from build123d import *

# Parameters (mm, degrees)
F1_DEPTH = 3
F2_DEPTH = 22.5
F0_W     = 13.580743
F0_H     = 20.673372
F0_R     = 1.5
F3_DEPTH = 5


with BuildPart() as f1:
    # F0 (on Front) → F1 (new body)
    with BuildSketch(Plane.XZ):
        Polygon((26.088619, 25.064645), (26.088619, 26.396385), (-26.088619, 26.396385), (-26.088619, 25.064645), (-26.088619, -25.064645), (26.088619, -25.064645), align=None)
    extrude(amount=F1_DEPTH)

    # F0 (on Front) → F2 (join)
    with BuildSketch(Plane.XZ):
        Polygon((-27.5, -26.396385), (27.5, -26.396385), (27.5, -10.336686), (27.5, 10.336686), (27.5, 26.396385), (26.088619, 26.396385), (26.088619, 25.064645), (26.088619, -25.064645), (-26.088619, -25.064645), (-26.088619, 25.064645), (-26.088619, 26.396385), (-27.5, 26.396385), (-27.5, 10.336686), (-27.5, -10.336686), align=None)
    extrude(amount=F2_DEPTH)

    # F0 (on Front) → F3 (join)
    with BuildSketch(Plane.XZ):
        with Locations((-34.290371, 0)):
            Rectangle(F0_W, F0_H)
        with Locations((-34.290372, 0)):
            Circle(F0_R, mode=Mode.SUBTRACT)
        with Locations((34.290371, 0)):
            Rectangle(F0_W, F0_H)
        with Locations((34.290372, 0)):
            Circle(F0_R, mode=Mode.SUBTRACT)
    extrude(amount=F3_DEPTH)


solid = f1.part
Verification items for the finished model (mm, model axes). A direction names the side the tool comes from. Round coordinates to 2 decimals unless told otherwise and drop trailing zeros. Loops run counter-clockwise (first coordinate to the right, second up) from the corner with the lowest first, then second, coordinate; pieces in that order, holes last. Notation, with made-up numbers: (76.5, -14) - (89.5, -14) arc R31 cw to (89.5, 12) - close; hole circle Ø2 at (54, 69). An arc over 180 degrees is marked (long way). Use one line per item in the form item = value.
1. Access from +Z, -Z, +X, -X, +Y, -Y to the whole of each face (thin tool, end or side, straight path). Record for faces 4 (the flat face through (26.089, -13, 1)), 5 (the flat face through (34, -2, 10.337)), 6 (the flat face through (34, -5, 2)), 7 (the flat face through (-34, -2, 10.337)), 8 (the flat face through (-34, -2, -10.337)).
A:
face_4 = +Z, -Y
face_5 = +Z, +X, +Y, -Y
face_6 = +Z, -Z, +X, -Y
face_7 = +Z, -X, +Y, -Y
face_8 = -Z, -X, +Y, -Y
2. Section check C-C on x = 24. Record the cut outline in (y, z).
A:
outline = (-22.5, -26.4) - (0, -26.4) - (0, 26.4) - (-3, 26.4) - (-3, -25.06) - (-22.5, -25.06) - close
3. Section check A-A on z = 0. Record the cut outline in (x, y).
A:
outline = (-41.08, -5) - (-35.79, -5) - (-35.79, 0) - (-41.08, 0) - close; (-32.79, -5) - (-27.5, -5) - (-27.5, -22.5) - (-26.09, -22.5) - (-26.09, -3) - (26.09, -3) - (26.09, -22.5) - (27.5, -22.5) - (27.5, -5) - (32.79, -5) - (32.79, 0) - (-32.79, 0) - close; (35.79, -5) - (41.08, -5) - (41.08, 0) - (35.79, 0) - close
4. Scan lines: probe 1 along X at (y, z) = (-19.75, 16); probe 2 along X at (y, z) = (-2.75, 16); probe 3 along Z at (x, y) = (1.5, -18.5). Record each from-to range of solid material in increasing order.
A:
probe_1 = -27.5 to -26.09, 26.09 to 27.5
probe_2 = -27.5 to 27.5
probe_3 = -26.4 to -25.06
5. Section check D-D on z = 5.5. Record the cut outline in (x, y), and give its area (3 significant figures).
A:
outline = (-41.08, -5) - (-27.5, -5) - (-27.5, -22.5) - (-26.09, -22.5) - (-26.09, -3) - (26.09, -3) - (26.09, -22.5) - (27.5, -22.5) - (27.5, -5) - (41.08, -5) - (41.08, 0) - (-41.08, 0) - close
area = 356 mm²
6. Gauge pin test, flat ends, axial feed: pin 1 Ø8 at (y, z) = (-16, 13.5) entering from -X; pin 2 Ø4 at (x, y) = (-33.5, -3) entering from -Z; pin 3 Ø11 at (x, z) = (37, 1) entering from -Y; pin 4 Ø1.8 at (x, z) = (34.29, 0) entering from -Y. Record the tip position at first contact, or that the pin passes through.
A:
pin_1 = -27.5
pin_2 = -10.34
pin_3 = -5
pin_4 = through
7. Section check B-B on y = -12. Record the cut outline in (x, z), and give its area (3 significant figures).
A:
outline = (-27.5, -26.4) - (27.5, -26.4) - (27.5, 26.4) - (26.09, 26.4) - (26.09, -25.06) - (-26.09, -25.06) - (-26.09, 26.4) - (-27.5, 26.4) - close
area = 219 mm²
8. Draft check along X on faces 1 (the flat face through (0, -13, -25.065)), 2 (the flat face through (34, -2, -10.337)), 3 (the flat face through (41.081, -2, 0)). Enter one of: pulls with the +X half, pulls with the -X half, needs draft (parallel to the pull), parting line crosses it, or undercut.
A:
face_1 = undercut
face_2 = needs draft
face_3 = pulls with the +X half
